Solid Edge part; units mm, degrees
sketch "Sketch1" plane through (0, 0, 16.7632) normal (0, 0, 1) x (1, 0, 0)
  circle A0 centre (-30.146, 20) radius 1.7
  circle A1 centre (30.146, 20) radius 1.7
  line L0 (-27.646, 31) -> (29.8105, 31)
  arc A2 (29.8105, 31) -> (36.8105, 24) centre (29.8105, 24) cw
  line L1 (36.8105, 24) -> (36.8105, 16)
  arc A3 (29.8105, 9) -> (36.8105, 16) centre (29.8105, 16) ccw
  line L2 (29.8105, 9) -> (17, 9)
  line L3 (17, 18.5) -> (17, 9)
  line L4 (17, 21.5) -> (17, 18.5)
  line L5 (8.3666, 21.5) -> (17, 21.5)
  arc A4 (-8.3666, 21.5) -> (8.3666, 21.5) centre (0, 20) cw
  line L6 (-15.5, 21.5) -> (-8.3666, 21.5)
  line L7 (-8.3666, 18.5) -> (-15.5, 18.5)
  line L8 (15.5, 18.5) -> (8.3666, 18.5)
  line L9 (15.5, 18.5) -> (15.5, 9)
  line L10 (15.5, 9) -> (-27.646, 9)
  arc A5 (-34.646, 16) -> (-27.646, 9) centre (-27.646, 16) ccw
  line L11 (-34.646, 16) -> (-34.646, 24)
  arc A6 (-34.646, 24) -> (-27.646, 31) centre (-27.646, 24) cw
  arc A7 (-15.5, 21.5) -> (-15.5, 18.5) centre (-15.5, 20) ccw
  arc A8 (-8.3666, 18.5) -> (8.3666, 18.5) centre (0, 20) ccw
extrude "ExtrudedProtrusion_1" add sketch "Sketch1" along normal blind 10
sketch "Sketch2" plane through (-6.073, 9, 21.7632) normal (0, -1, 0) x (1, 0, 0)
  circle A0 centre (-15.6919, -5) radius 5.5
extrude "Cutout1" cut sketch "Sketch2" against normal up to next
sketch "Sketch3" plane through (-6.073, 9, 21.7632) normal (0, -1, 0) x (1, 0, 0)
  line L0 (15.8501, -1.1809) -> (17.073, -2.4472)
  line L1 (17.073, -2.4472) -> (18.2959, -1.1809)
  arc A0 (15.8501, -1.1809) -> (18.2959, -1.1809) centre (17.073, 0) cw
extrude "Cutout2" cut sketch "Sketch3" against normal through all
sketch "Sketch4" plane through (1.0823, 20, 26.7632) normal (0, 0, 1) x (1, 0, 0)
  circle A0 centre (-11.0823, 0) radius 3
extrude "Cutout3" cut sketch "Sketch4" against normal through all
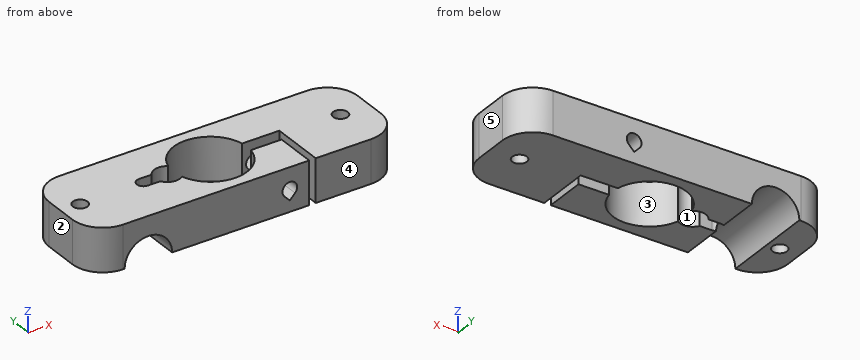
CAD build for the part. Positions are in the model's coordinates, mm. Face numbers are marked on the shaded views. A direction names the side the tool comes from. Give positions to 0.01 mm unless a question says otherwise; leave off trailing zeros. Order: outer loops, then holes, each group sorted by start corner. A loop starts at its lowest first (then second) coordinate and runs counter-clockwise, first axis right, second up. Notation, with made-up numbers: M 50.25,59.5 L 76.25,59.5 A32 cw 76.25,87.5 Z; hole C 87,9.25 d8. An arc over 180 degrees is marked long. Put each result on its own line as item: value. Start each with the question number.
(1) Flat gauge pin, fed straight in: pin 1 Ø3 at (x, y) = (30.146, 20) entering from -Z. Where does the tip first touch, or does it go through?
(2) Saw through at B-B, the plane y = 10.5. Write the cut outline in (x, z), then the cut area to 3 significant figures.
(3) Mould opens along Y. For the marked faces 3, 4 and 5 say: +Y half, -Y half, draft (parallel to the pull), parting line (faces both ways), or undercut.
(4) Drill centre lines: line 1 along X through (y, z) = (16, 19.25); line 2 along Y through (x, z) = (0.5, 25.25); line 3 along Y through (x, z) = (7.5, 20.75). Where is each one in solid material? Low to high.
(5) Which spindle directions (+Z, -Z, +X, -X, +Y, -Y) get a long thin tool onto all of the face, cutting with end or side? Do the marked faces 1 and 2. Say none if no direction does.
(6) Saw through at A-A, the plane y = 13.5. Write the cut outline in (x, z).
(7) Saw through at D-D, the plane x = -11.5. Write the cut outline in (y, z).
(8) Saw through at C-C, the plane z = 26. Write the cut outline in (x, y).
Check result:
1. pin 1: passes through
2. outline: M -31.98,16.76 L -27.26,16.76 A5.5 cw -16.26,16.76 L 15.5,16.76 L 15.5,26.76 L -31.98,26.76 Z; M 17,16.76 L 34.14,16.76 L 34.14,26.76 L 17,26.76 Z; hole M 9.78,20.58 L 11,19.32 L 12.22,20.58 A1.7 ccw long Z
2. area: 589 mm2
3. face 3: undercut
3. face 4: -Y half
3. face 5: draft
4. line 1: x = -34.65 to -26.67, -16.86 to -7.5, 7.5 to 15.5, 17 to 36.81
4. line 2: y = 9 to 11.51, 28.49 to 31
4. line 3: y = 9 to 16, 24 to 31
5. face 1: +Z, -Z
5. face 2: +Z, -Z, -X, +Y, -Y
6. outline: M -34.18,16.76 L -27.26,16.76 A5.5 cw -16.26,16.76 L -5.48,16.76 L -5.48,26.76 L -34.18,26.76 Z; M 5.48,16.76 L 15.5,16.76 L 15.5,26.76 L 5.48,26.76 Z; M 17,16.76 L 36.35,16.76 L 36.35,26.76 L 17,26.76 Z; hole M 9.78,20.58 L 11,19.32 L 12.22,20.58 A1.7 ccw long Z
7. outline: M 9,16.76 L 17.4,16.76 L 17.4,26.76 L 9,26.76 Z; M 22.6,16.76 L 31,16.76 L 31,26.76 L 22.6,26.76 Z
8. outline: M -34.65,16 A7 ccw -27.65,9 L 15.5,9 L 15.5,18.5 L 8.37,18.5 A8.5 cw -8.16,17.63 A3 cw -12.6,18.5 L -15.5,18.5 A1.5 cw -15.5,21.5 L -12.6,21.5 A3 cw -8.16,22.37 A8.5 cw 8.37,21.5 L 17,21.5 L 17,9 L 29.81,9 A7 ccw 36.81,16 L 36.81,24 A7 ccw 29.81,31 L -27.65,31 A7 ccw -34.65,24 Z; hole C -30.15,20 d3.4; hole C 30.15,20 d3.4
